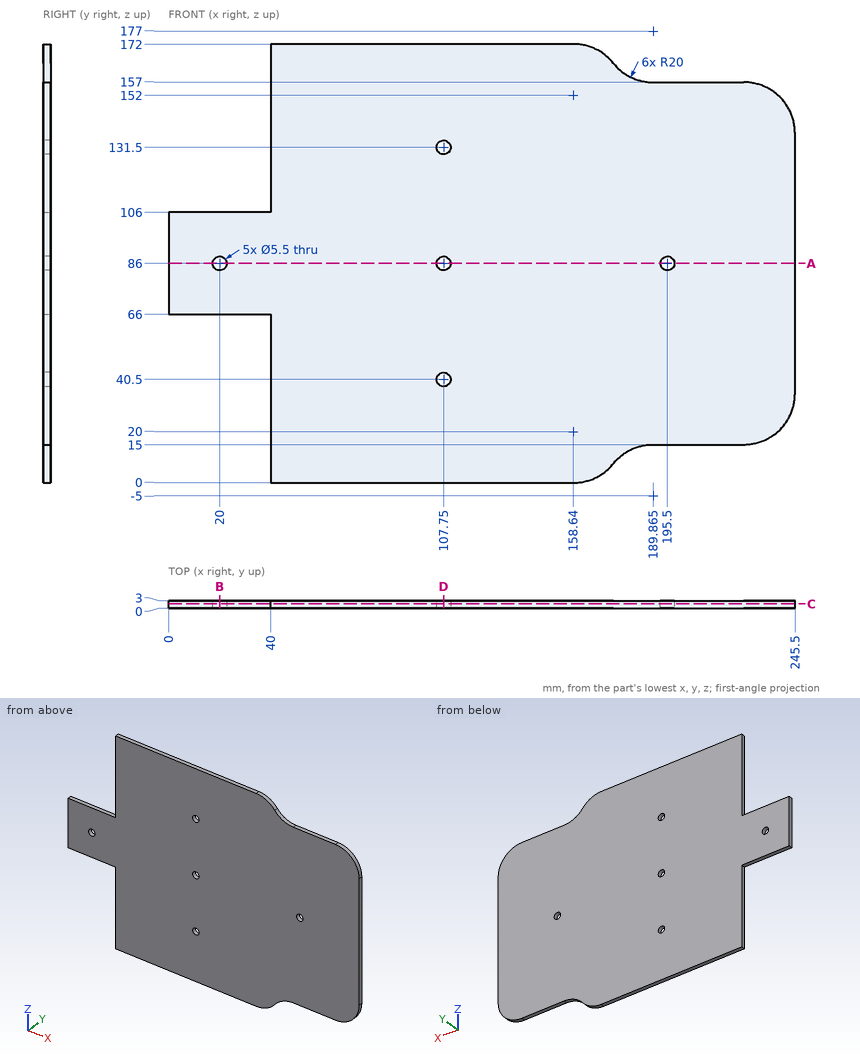
Geometry: see drawing. Coordinates: mm, zero at the bounding-box minimum. Coordinates: 2 decimals unless noted, no trailing zeros. Order: outer loops, then holes, each group sorted by start corner. A loop starts at its lowest first (then second) coordinate and runs counter-clockwise, first axis right, second up. Notation, with made-up numbers: (19.25, 70.25) - (29.25, 70.25) arc R11 cw to (29.25, 74.25) - close; hole circle Ø5 at (-13, -5.75). An arc over 180 degrees is marked (long way). Write each question's results on one line, items separated by ' | '.
1) Section C-C, the plane y = 1.85. State how many separate pieces and enclosed holes the cut face has, plus the area to 3 significant figures.
Results list:
separate pieces: 1 | enclosed holes: 5 | area: 34,500 mm^2
2) Section B-B, the plane x = 20. Return loops of the section in (y, z), plus the area to 4 significant figures.
Results list:
outline: (0, 66) - (3, 66) - (3, 83.25) - (0, 83.25) - close; (0, 88.75) - (3, 88.75) - (3, 106) - (0, 106) - close | area: 103.5 mm^2
3) Section A-A, the plane z = 86. Return loops of the section in (x, y), plus the area to 3 significant figures.
Results list:
outline: (0, 0) - (17.25, 0) - (17.25, 3) - (0, 3) - close; (22.75, 0) - (105, 0) - (105, 3) - (22.75, 3) - close; (110.5, 0) - (192.75, 0) - (192.75, 3) - (110.5, 3) - close; (198.25, 0) - (245.5, 0) - (245.5, 3) - (198.25, 3) - close | area: 687 mm^2
4) Section D-D, the plane x = 107.75. Return loops of the section in (y, z).
Results list:
outline: (0, 0) - (3, 0) - (3, 37.75) - (0, 37.75) - close; (0, 43.25) - (3, 43.25) - (3, 83.25) - (0, 83.25) - close; (0, 88.75) - (3, 88.75) - (3, 128.75) - (0, 128.75) - close; (0, 134.25) - (3, 134.25) - (3, 172) - (0, 172) - close
5) Line query: line 1 (Z direction, x = 107.75, y = 1.9); line 2 (Z direction, x = 20, y = 2.15); line 3 (Z direction, x = 195.5, y = 2.35). Output: solid intervals per line, ascending. Write a range as from..to.
Results list:
line 1: 0..37.75, 43.25..83.25, 88.75..128.75, 134.25..172 | line 2: 66..83.25, 88.75..106 | line 3: 15..83.25, 88.75..157
6) Pin query (flat end, axial travel): pin 1 (3.5 mm diameter, centred on x = 107.75, z = 131.5, fed in from +Y); pin 2 (0.9 mm diameter, centred on x = 200, y = 1, fed in from -Z); pin 3 (1.5 mm diameter, centred on x = 16.5, y = 1, fed in from -Z); pin 4 (1.5 mm diameter, centred on x = 208, y = 1.5, fed in from +Z). Return the tip coordinate at first contact, or that it passes through.
Results list:
pin 1: through | pin 2: z = 15 | pin 3: z = 66 | pin 4: z = 157
